```python
from build123d import *

# Parameters (mm, degrees)
BOSS_EXTRU_1_DEPTH      = 28
ENL_V_MAT_EXTRU_1_DEPTH = 40
ESQUISSE3_W             = 33
ESQUISSE3_H             = 20
ENL_V_MAT_EXTRU_2_DEPTH = 20
D_GAGEMENT_M41_D        = 4.4
D_GAGEMENT_M41_DEPTH    = 5
D_GAGEMENT_M42_D        = 4.4
D_GAGEMENT_M43_D        = 4.4
D_GAGEMENT_M43_DEPTH    = 5
ESQUISSE13_W            = 5
ESQUISSE13_H            = 12
ENL_V_MAT_EXTRU_4_DEPTH = 10


with BuildPart() as part:
    # Esquisse1 → Boss.-Extru.1 (new body)
    with BuildSketch(Plane.XY):
        Polygon((0, 0), (64, 0), (64, -24), (24, -24), (24, -44), (0, -44), align=None)
    extrude(amount=BOSS_EXTRU_1_DEPTH)

    # Esquisse2 → Enlèv. mat.-Extru.1 (cut)
    with BuildSketch(Plane.XZ.offset(44)):
        Polygon((24, 24), (17, 24), (17, 21.5), (11, 21.5), (11, 24), (4, 24), (4, 4), (11, 4), (11, 6.5), (17, 6.5), (17, 4), (24, 4), align=None)
    extrude(amount=-ENL_V_MAT_EXTRU_1_DEPTH, mode=Mode.SUBTRACT)

    # Esquisse3 → Enlèv. mat.-Extru.2 (cut)
    with BuildSketch(Plane.XZ.offset(24)):
        with Locations((47.5, 14)):
            Rectangle(ESQUISSE3_W, ESQUISSE3_H)
    extrude(amount=-ENL_V_MAT_EXTRU_2_DEPTH, mode=Mode.SUBTRACT)

    # Dégagement M41
    with Locations(Plane.ZY):
        with Locations((14, -15.5), (14, -30.5)):
            Hole(D_GAGEMENT_M41_D / 2, depth=D_GAGEMENT_M41_DEPTH)

    # Dégagement M42 (through all)
    with Locations(Plane.XY.offset(28)):
        with Locations((39, -14)):
            Hole(D_GAGEMENT_M42_D / 2)

    # Dégagement M43
    with Locations(Plane(origin=(0, 0, 0), x_dir=(1, 0, 0), z_dir=(0, 1, 0))):
        with Locations((49, -14)):
            Hole(D_GAGEMENT_M43_D / 2, depth=D_GAGEMENT_M43_DEPTH)

    # Esquisse13 → Enlèv. mat.-Extru.4 (cut)
    with BuildSketch(Plane(origin=(0, 0, 0), x_dir=(1, 0, 0), z_dir=(0, 1, 0))):
        with Locations((7.5, -14)):
            Rectangle(ESQUISSE13_W, ESQUISSE13_H)
    extrude(amount=-ENL_V_MAT_EXTRU_4_DEPTH, mode=Mode.SUBTRACT)


solid = part.part
```
Can you work these out from the model? Positions are in its coordinate system, mm. A direction names the side the tool comes from. Round coordinates to 2 decimals unless told otherwise and drop trailing zeros. Loops run counter-clockwise (first coordinate to the right, second up) from the corner with the lowest first, then second, coordinate; pieces in that order, holes last. Notation, with made-up numbers: M 69,74.25 L 110,74.25 A23 cw 110,86.25 Z; hole C 72.5,60.25 d8. An arc over 180 degrees is marked long. Write item = value, one per line. Start each with the question number.
(1) I'm going to push flat-ended pins straight in: P1, Ø2, axis at y = -30.5, z = 26, coming from the +X side; P2, Ø5, axis at x = 35, z = 23.5, coming from the -Y side; P3, Ø4, axis at x = 33.5, z = 6.5, coming from the -Y side. Where does each tip first touch, or does it pass through?
(2) Suppose I cut it at D-D on y = -14. Give the number of separate pieces and of enclosed holes in the cut face, plus the area to 3 significant figures.
(3) If we mould it in two halves opening along X, with no side actions, what happens to faces 4 (the face through (47, -4, 12)), 5 (the face through (10, -2, 14)), 6 (the face through (7, -2, 8)), 7 (the face through (31, -14, 14))? For each: released by +X, released by -X, zero draft, split by the parting line, or undercut.
(4) Suppose I cut it at C-C on y = -30.5. Write out the boundary of the cut face in (x, z).
(5) I need wall thicknesses on line 1 along X through (y, z) = (-2.95, 14); line 2 along Y through (x, z) = (39, 25.75); line 3 along Z through (x, y) = (14, -11.5). Which ranges of each line are inside material? Lowest first, please.
(6) Which directions (+Z, -Z, +X, -X, +Y, -Y) give clear straight access to the entire face, cutting with the end or side of a thin tool? Please do faces 1 (the face through (24, -34, 2)), 2 (the face through (17, -24, 23)), 3 (the face through (41.198, -13.903, 25.972)).
(7) Suppose I cut it at A-A on x = 39. Write out the boundary of the cut face in (y, z).
(8) Suppose I cut it at B-B on z = 3. Write out the boundary of the cut face in (x, y), plus the area to 3 significant figures.
Answer block:
q1.P1 = 24
q1.P2 = -24
q1.P3 = -4
q2.separate_pieces = 3
q2.enclosed_holes = 0
q2.area = 714 mm²
q3.face_4 = zero draft
q3.face_5 = undercut
q3.face_6 = undercut
q3.face_7 = released by +X
q4.outline = M 0,0 L 24,0 L 24,4 L 17,4 L 17,6.5 L 11,6.5 L 11,4 L 4,4 L 4,11.8 L 0,11.8 Z; M 0,16.2 L 4,16.2 L 4,24 L 11,24 L 11,21.5 L 17,21.5 L 17,24 L 24,24 L 24,28 L 0,28 Z
q5.line_1 = 0 to 5, 10 to 46.8, 51.2 to 64
q5.line_2 = -24 to -16.2, -11.8 to 0
q5.line_3 = 0 to 6.5, 21.5 to 28
q6.face_1 = +Z, -Z, +X, -Y
q6.face_2 = -Y
q6.face_3 = +Z, -Z
q7.outline = M -24,0 L -16.2,0 L -16.2,4 L -24,4 Z; M -24,24 L -16.2,24 L -16.2,28 L -24,28 Z; M -11.8,0 L 0,0 L 0,28 L -11.8,28 L -11.8,24 L -4,24 L -4,4 L -11.8,4 Z
q8.outline = M 0,-44 L 24,-44 L 24,-24 L 64,-24 L 64,0 L 0,0 Z; hole C 39,-14 d4.4
q8.area = 2,000 mm²
